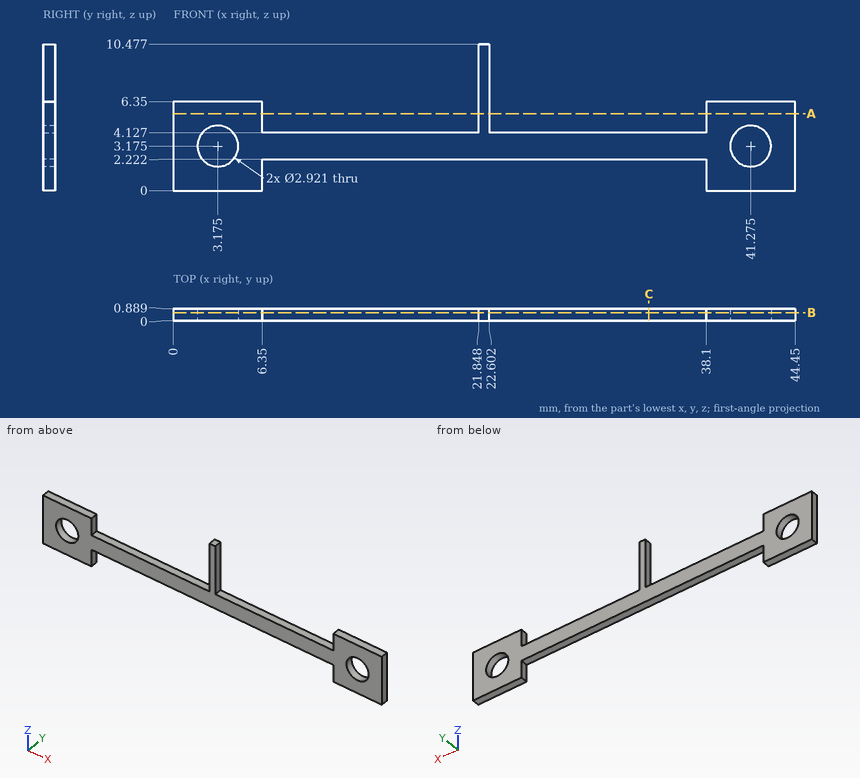
Study the drawing (mm; zero at the part's minimum x, y, z) and answer. Give positions to 0.01 mm unless a question says otherwise; leave off trailing zeros. Write each loop counter-clockwise with the first axis right and the second up, starting at its lowest first coordinate (ties: lowest second). Pieces come first, ordered by that corner, then holes. Notation, with made-up numbers: (-12.75, -16) -> (35.25, -16) arc R35 ccw to (35.25, 18) -> close; hole circle Ø4 at (-38.5, -35). An arc over 180 degrees is marked (long way). Answer in a Markdown table with one row per item.
1) Section C-C on x = 34 is taken. Give the vertices of the cut face in (y, z).
Results list:
| item | result |
|---|---|
| outline | (0, 2.22) -> (0.89, 2.22) -> (0.89, 4.13) -> (0, 4.13) -> close |
2) This flat-tipped pin is pushed along its axis until it touches: pin 1 Ø6 at (x, z) = (38, 7) entering from -Y. Where does it stop, or does it pass through?
Results list:
| item | result |
|---|---|
| pin 1 | y = 0 |
3) Section B-B on y = 0.6 is taken. Count the separate pieces of the cut face and the enclosed holes in it.
Results list:
| item | result |
|---|---|
| separate pieces | 1 |
| enclosed holes | 2 |
4) Straight lines are drawn through the part: line 1 (X direction, y = 0.3, z = 6); line 2 (X direction, y = 0.25, z = 0.75); line 3 (X direction, y = 0.75, z = 4). For each, find the intervals that lie inside material, in ascending order. Write a range as [from, to].
Results list:
| item | result |
|---|---|
| line 1 | [0, 6.35], [21.85, 22.6], [38.1, 44.45] |
| line 2 | [0, 6.35], [38.1, 44.45] |
| line 3 | [0, 1.97], [4.38, 40.07], [42.48, 44.45] |
5) Section A-A on z = 5.5 is taken. Give the vertices of the cut face in (x, y).
Results list:
| item | result |
|---|---|
| outline | (0, 0) -> (6.35, 0) -> (6.35, 0.89) -> (0, 0.89) -> close; (21.85, 0) -> (22.6, 0) -> (22.6, 0.89) -> (21.85, 0.89) -> close; (38.1, 0) -> (44.45, 0) -> (44.45, 0.89) -> (38.1, 0.89) -> close |
